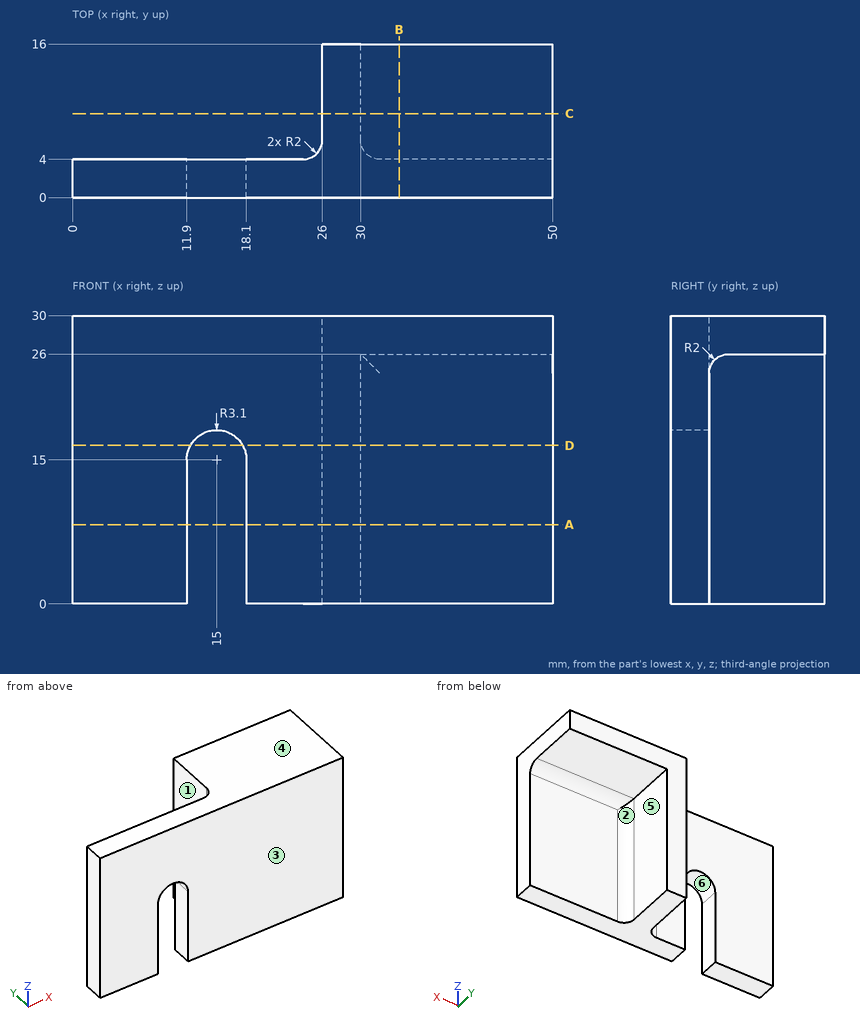
Part print with two shaded views. Sizes in mm from the minimum x, y, z corner. A direction names the side the tool comes from. Coordinates: 2 decimals unless noted, no trailing zeros. Write each loop counter-clockwise with the first axis right and the second up, starting at its lowest first coordinate (ties: lowest second). Pieces come first, ordered by that corner, then holes. Notation, with made-up numbers: (50, -5.75) - (91, -5.75) arc R17 ccw to (91, 12.25) - close; hole circle Ø9 at (28, -31.5). An arc over 180 degrees is marked (long way). One line per item, written item: value. Start each with the question number.
1. Flat gauge pins, fed straight in: pin 1 (1.5 mm diameter, centred on y = 10, z = 22.5, fed in from +X); pin 2 (3 mm diameter, centred on x = 35, y = 12, fed in from -Z); pin 3 (14.5 mm diameter, centred on x = 42.5, z = 15, fed in from +Y). Where does each tip first touch, or does it go through?
2. Slice it at C-C (y = 8.75). Write the cut outline in (x, z), plus the area to 3 significant figures.
3. Slice it at D-D (z = 16.5). Write the cut outline in (x, y), plus the area to 3 significant figures.
4. Slice it at A-A (z = 8.25). Write the cut outline in (x, y), plus the area to 3 significant figures.
5. Slice it at B-B (x = 34). Write the cut outline in (y, z), plus the area to 3 significant figures.
6. Tool access for the marked faces 1, 2 and 3: list every direction of +Z, -Z, +X, -X, +Y, -Y with a clear straight run to the whole face (end or side of a thin tool).
7. Probe line 1 (X direction, y = 1, z = 12.25); line 2 (Z direction, x = 15, y = 3.5); line 3 (X direction, y = 14.75, z = 25). List the from-to ranges inside material, lowest first. Write a range as from..to.
8. Mould opens along X. For the marked faces 4, 5 and 6 say: released by +X, released by -X, zero draft, split by the parting line, or undercut.
Answers below:
1. pin 1: stops at x = 30
1. pin 2: stops at z = 26
1. pin 3: stops at y = 4
2. outline: (26, 0) - (30, 0) - (30, 26) - (50, 26) - (50, 30) - (26, 30) - close
2. area: 200 mm^2
3. outline: (0, 0) - (12.29, 0) - (12.29, 4) - (0, 4) - close; (17.71, 0) - (50, 0) - (50, 4) - (32, 4) arc R2 cw to (30, 6) - (30, 16) - (26, 16) - (26, 6) arc R2 cw to (24, 4) - (17.71, 4) - close
3. area: 228 mm^2
4. outline: (0, 0) - (11.9, 0) - (11.9, 4) - (0, 4) - close; (18.1, 0) - (50, 0) - (50, 4) - (32, 4) arc R2 cw to (30, 6) - (30, 16) - (26, 16) - (26, 6) arc R2 cw to (24, 4) - (18.1, 4) - close
4. area: 225 mm^2
5. outline: (0, 0) - (4, 0) - (4, 24) arc R2 cw to (6, 26) - (16, 26) - (16, 30) - (0, 30) - close
5. area: 169 mm^2
6. face 1: +Z, -Z, -X, +Y
6. face 2: -Z, +X, +Y
6. face 3: +Z, -Z, +X, -X, -Y
7. line 1: x = 0..11.9, 18.1..50
7. line 2: z = 18.1..30
7. line 3: x = 26..30
8. face 4: zero draft
8. face 5: released by +X
8. face 6: undercut
